Source: CAD feature listing. Evaluate the final solid. Frame: model axes, mm. Face numbers are marked on the shaded views. A direction names the side the tool comes from. Give positions to 0.01 mm unless a question says otherwise; leave off trailing zeros. Write each loop counter-clockwise with the first axis right and the second up, starting at its lowest first coordinate (ties: lowest second). Pieces come first, ordered by that corner, then holes.
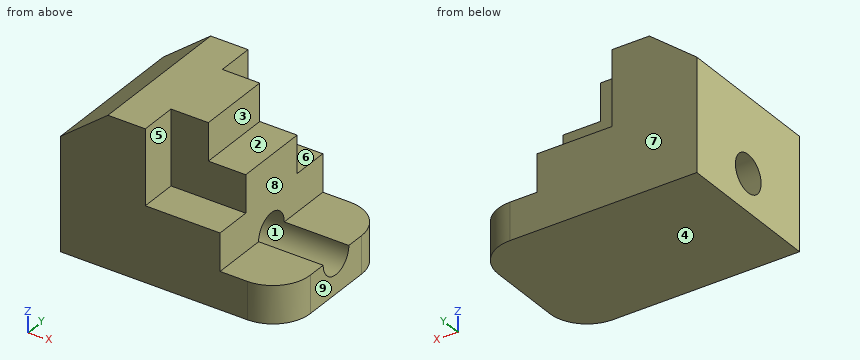
```python
from build123d import *

# Parameters (mm, degrees)
F1_DEPTH = 25.4
F2_R     = 6.35
F3_DEPTH = 54.256924135
F5_DEPTH = 76.201
F7_DEPTH = 12.7
F9_DEPTH = 12.7
F10_R    = 12.7


with BuildPart() as f1:
    # F0 (on Front) → F1 (new body, symmetric)
    with BuildSketch(Plane.XZ):
        Polygon((0, 38.1), (0, 0), (76.2, 0), (76.2, 12.7), (54.255924135, 12.7), (54.255924135, 38.1), (41.555924135, 38.1), (41.555924135, 50.8), (16.155924135, 50.8), align=None)
    extrude(amount=F1_DEPTH, both=True)

    # F2 (on face) → F3 (cut, through all)
    with BuildSketch(Plane.YZ.offset(54.255924135)):
        with Locations((0, 12.7)):
            Circle(F2_R)
    extrude(amount=-F3_DEPTH, mode=Mode.SUBTRACT)

    # F4 (on face) → F5 (cut, through all)
    with BuildSketch(Plane.YZ.offset(76.2)):
        with BuildLine():
            ThreePointArc((-6.35, 12.7), (0, 6.35), (6.35, 12.7))
            Line((6.35, 12.7), (-6.35, 12.7))
        make_face()
    extrude(amount=-F5_DEPTH, mode=Mode.SUBTRACT)

    # F6 (on face) → F7 (cut)
    with BuildSketch(Plane.XZ.offset(25.4)):
        Polygon((41.555924135, 50.8), (28.855924135, 50.8), (28.855924135, 25.4), (54.255924135, 25.4), (54.255924135, 38.1), (41.555924135, 38.1), align=None)
    extrude(amount=-F7_DEPTH, mode=Mode.SUBTRACT)

    # F8 (on face) → F9 (cut)
    with BuildSketch(Plane(origin=(0, 25.4, 0), x_dir=(-1, 0, 0), z_dir=(0, 1, 0))):
        Polygon((-28.855924135, 25.4), (-28.855924135, 50.8), (-41.555924135, 50.8), (-41.555924135, 38.1), (-54.255924135, 38.1), (-54.255924135, 25.4), align=None)
    extrude(amount=-F9_DEPTH, mode=Mode.SUBTRACT)

    # F10
    f10_edges = [f1.edges().sort_by_distance(p)[0] for p in [
        (76.2, 25.4, 6.35),
        (76.2, -25.4, 6.35),
    ]]
    fillet(f10_edges, radius=F10_R)


solid = f1.part
```
1. Line query: probe 1 along Z at (x, y) = (45, 0); probe 2 along Z at (x, y) = (36.5, 0); probe 3 along Z at (x, y) = (50.5, 11.5). Output: solid intervals per line, ascending.
2. Pull-direction query (Z, two-part tool) for the marked faces 1, 2, 3 and 4; classes: pulls with the +Z half, pulls with the -Z half, needs draft (parallel to the pull), parting line crosses it, or undercut.
3. Section query D-D (y = -7.5). Return loops of the section in (x, z), plus the area to 3 significant figures.
4. Access query for the marked faces 5, 6, 7, 8 and 9. Directions: +Z, -Z, +X, -X, +Y, -Y. A direction counts if a zero-diameter tool reaches every point of the face in a straight line with its end or side. Return the directions, or none.
5. Pin query (flat end, axial travel): P1, Ø7.5, axis at y = 4, z = 21, coming from the +X side; P2, Ø10, axis at x = 37, y = -22, coming from the +Z side; P3, Ø10, axis at y = -22, z = 42, coming from the +X side. Return the tip coordinate at first contact, or that it passes through.
6. Section query C-C (z = 9). Return loops of the section in (x, y), plus the area to 3 significant figures.
7. Section query A-A (y = 0). Return loops of the section in (x, z), plus the area to 3 significant figures.
8. Section query B-B (x = 24). Return loops of the section in (y, z).
The answers:
1. probe 1: z = 0 to 6.35, 19.05 to 38.1
1. probe 2: z = 0 to 6.35, 19.05 to 50.8
1. probe 3: z = 0 to 38.1
2. face 1: undercut
2. face 2: pulls with the +Z half
2. face 3: needs draft
2. face 4: pulls with the -Z half
3. outline: (0, 0) - (76.2, 0) - (76.2, 12.7) - (54.26, 12.7) - (54.26, 38.1) - (41.56, 38.1) - (41.56, 50.8) - (16.16, 50.8) - (0, 38.1) - close
3. area: 2,770 mm2
4. face 5: +Z, +X, -Y
4. face 6: +Z, +X, +Y
4. face 7: +Z, -Z, +X, -X, +Y
4. face 8: +Z, +X, +Y, -Y
4. face 9: +Z, -Z, +X, +Y, -Y
5. P1: stops at x = 54.26
5. P2: stops at z = 25.4
5. P3: stops at x = 28.86
6. outline: (0, -25.4) - (63.5, -25.4) arc R12.7 ccw to (76.2, -12.7) - (76.2, -5.16) - (0, -5.16) - close; (0, 5.16) - (76.2, 5.16) - (76.2, 12.7) arc R12.7 ccw to (63.5, 25.4) - (0, 25.4) - close
6. area: 3,020 mm2
7. outline: (0, 0) - (76.2, 0) - (76.2, 6.35) - (0, 6.35) - close; (0, 19.05) - (54.26, 19.05) - (54.26, 38.1) - (41.56, 38.1) - (41.56, 50.8) - (16.16, 50.8) - (0, 38.1) - close
7. area: 1,940 mm2
8. outline: (-25.4, 0) - (25.4, 0) - (25.4, 50.8) - (-25.4, 50.8) - close; hole circle Ø12.7 at (0, 12.7)
